The model under review builds one solid part; all positions refer to its coordinate system, in mm. Face numbers are marked on the shaded views. Round coordinates to 2 decimals unless told otherwise and drop trailing zeros. Order: outer loops, then holes, each group sorted by start corner. A loop starts at its lowest first (then second) coordinate and runs counter-clockwise, first axis right, second up. Notation, with made-up numbers: M 19,60 L 70,60 A12 ccw 70,82 Z; hole C 57,-27 d11. An arc over 180 degrees is marked long. Use a Markdown table: item, result. Add a question column.
1. To check wall thickness, follow probe 1 along X at (y, z) = (0.5, 1.6); probe 2 along Y at (x, z) = (-0.25, 0.4); probe 3 along Y at (x, z) = (-0.6, 0.35). State the ranges of each line that lie inside material, in increasing order.
2. Consider section A-A on z = 1.2. State the section outline as (x, y) points, then the cut area to 3 significant figures.
3. The part is to be moulded in two halves that separate along X. For the marked faces 1, 2 and 3, say which applies: +X half, -X half, draft (parallel to the pull), parting line (faces both ways), or undercut.
Autodesk Inventor part; units mm, degrees
ref_plane "YZ Plane" through (0, 0, 0) normal (1, 0, 0) x (0, 1, 0)
ref_plane "XZ Plane" through (0, 0, 0) normal (0, 1, 0) x (-1, 0, 0)
ref_plane "XY Plane" through (0, 0, 0) normal (0, 0, 1) x (1, 0, 0)
sketch "Náčrt1" plane through (0, 0, 0) normal (0, 0, 1) x (1, 0, 0)
  line L0 (2.75, -1.5877) -> (0, -3.1754)
  line L1 (0, -3.1754) -> (-2.75, -1.5877)
  line L2 (-2.75, -1.5877) -> (-2.75, 1.5877)
  line L3 (-2.75, 1.5877) -> (0, 3.1754)
  line L4 (0, 3.1754) -> (2.75, 1.5877)
  line L5 (2.75, 1.5877) -> (2.75, -1.5877)
  circle A0 centre (0, 0) radius 1.5
  point P0 (2.75, 0)
  dimension "d1" = 3
extrude "Vysunutí1" add sketch "Náčrt1" along normal blind 2.4
thread "Závit1"
sketch "Náčrt2" plane through (0, 0, 2.4) normal (0, 0, 1) x (1, 0, 0)
  circle A0 centre (0, 0) radius 2.75
extrude "Vysunutí2" cut sketch "Náčrt2" against normal through all draft 45 keep common part
sketch "Náčrt3" plane through (0, 0, 0) normal (0, 0, -1) x (-1, 0, 0)
  circle A0 centre (0, 0) radius 2.75
extrude "Vysunutí3" cut sketch "Náčrt3" against normal through all draft 45 keep common part
chamfer "Zkosení1" distance 0.2 angle 45 1 edges at (-1.5, 0, 2.4)
chamfer "Zkosení2" distance 0.2 angle 45 1 edges at (-1.5, 0, 0)
properties part number "Nut-M3" material "Ocel, vysokopevnostní, nízkolegovaná"
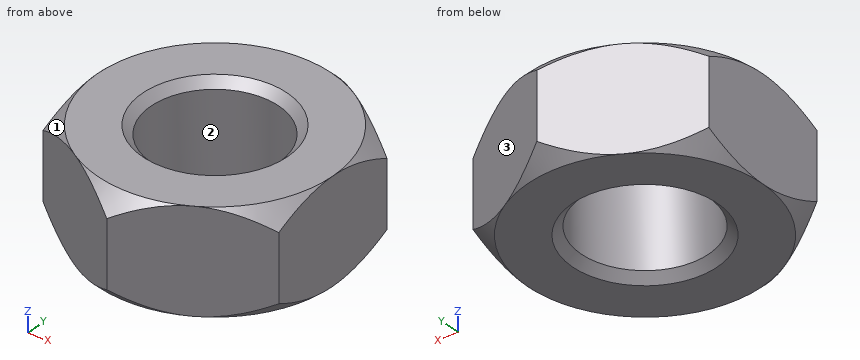
Answer block:
| question | item | result |
|---|---|---|
| 1 | probe 1 | -2.75 to -1.41, 1.41 to 2.75 |
| 1 | probe 2 | -3.03 to -1.48, 1.48 to 3.03 |
| 1 | probe 3 | -2.83 to -1.37, 1.37 to 2.83 |
| 2 | outline | M -2.75,-1.59 L 0,-3.18 L 2.75,-1.59 L 2.75,1.59 L 0,3.18 L -2.75,1.59 Z; hole C 0,0 d3 |
| 2 | area | 19.1 mm^2 |
| 3 | face 1 | -X half |
| 3 | face 2 | undercut |
| 3 | face 3 | +X half |
